Verification items for the finished model (mm, model axes). Face numbers are marked on the shaded views. A direction names the side the tool comes from. Round coordinates to 2 decimals unless told otherwise and drop trailing zeros. Order: outer loops, then holes, each group sorted by start corner. A loop starts at its lowest first (then second) coordinate and runs counter-clockwise, first axis right, second up. Notation, with made-up numbers: (54, 83) -> (81, 83) arc R30 ccw to (81, 113) -> close; hole circle Ø3 at (45.25, 49.25). An arc over 180 degrees is marked (long way). Put each result on its own line as item: value.
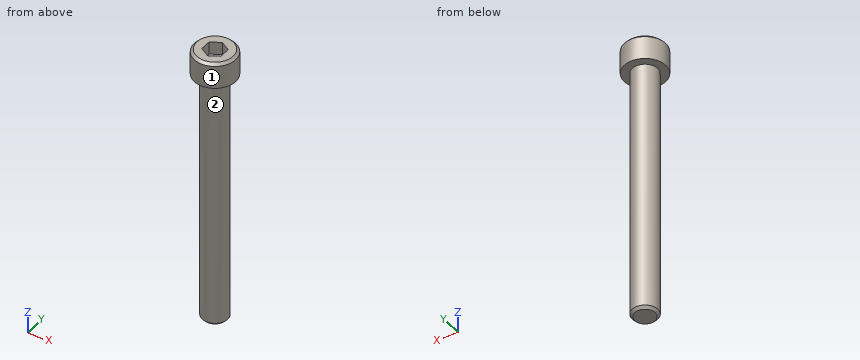
Autodesk Inventor part; units mm, degrees
ref_plane "YZ Plane" through (0, 0, 0) normal (1, 0, 0) x (0, 1, 0)
ref_plane "XZ Plane" through (0, 0, 0) normal (0, 1, 0) x (-1, 0, 0)
ref_plane "XY Plane" through (0, 0, 0) normal (0, 0, 1) x (1, 0, 0)
sketch "Sketch1" plane through (0, 0, 0) normal (0, 0, 1) x (1, 0, 0)
  circle A0 centre (0, 0) radius 4
  dimension "Diameter" = 8
extrude "Extrusion1" add sketch "Sketch1" along normal blind 80
sketch "Sketch2" plane through (0, 0, 80) normal (0, 0, 1) x (1, 0, 0)
  circle A0 centre (0, 0) radius 4
  circle A1 centre (0, 0) radius 6.5
  dimension "Head_Diameter" = 13
extrude "Extrusion2" add sketch "Sketch2" along normal blind 8 contours A0 | A1
sketch "Sketch3" plane through (0, 0, 88) normal (0, 0, 1) x (1, 0, 0)
  circle A0 centre (0, 0) radius 6.5
  circle A1 centre (0, 0) radius 3.4641 construction
  line L0 (0, 3.4641) -> (3, 1.7321)
  line L1 (3, -1.7321) -> (3, 1.7321)
  line L2 (0, 3.4641) -> (-3, 1.7321)
  line L3 (-3, -1.7321) -> (-3, 1.7321)
  line L4 (-3, -1.7321) -> (0, -3.4641)
  line L5 (3, -1.7321) -> (0, -3.4641)
  dimension "Hex_Width" = 6
extrude "Extrusion3" cut sketch "Sketch3" against normal blind 4 contours L0 L1 L5 L4 L3 L2
thread "Thread1"
chamfer "Chamfer1" distance 0.8 angle 45 2 edges at (-6.5, 0, 88) (-4, 0, 0)
equation "\"d9\" = ThreadLength"
equation "\"d12\" = Chamfer"
equation "\"ThreadLength\" = 28"
properties part number "SCREW,SOCKET HD,P,12.9,M8X1.25X80MM"
Item 1: Sectioned sample at A-A, the plane y = 0. Record the boundary of the cut face in (x, z).
Geometry check:
outline: (-6.5, 80) -> (-4, 80) -> (-4, 0.8) -> (-3.2, 0) -> (3.2, 0) -> (4, 0.8) -> (4, 80) -> (6.5, 80) -> (6.5, 87.2) -> (5.7, 88) -> (3, 88) -> (3, 84) -> (-3, 84) -> (-3, 88) -> (-5.7, 88) -> (-6.5, 87.2) -> close
Item 2: Sectioned sample at B-B, the plane z = 8.5. Record the boundary of the cut face in (x, y), then the cut area to 3 significant figures.
Geometry check:
outline: circle Ø8 at (0, 0)
area: 50.3 mm2
Item 3: Material ranges on line 1 along Z through (x, y) = (-3, -3.75); line 2 along Z through (x, y) = (0.75, 1); line 3 along X through (y, z) = (0.25, 83), recorded low to high.
Geometry check:
line 1: 80 to 88
line 2: 0 to 84
line 3: -6.5 to 6.5
Item 4: Tool access check on the marked faces 1 and 2. Record the directions out of +Z, -Z, +X, -X, +Y, -Y that give a thin tool (end or side, any length) a straight path to the whole face; none if there is none.
Geometry check:
face 1: +Z, -Z
face 2: -Z
Item 5: Depth check by flat-ended pin: pin 1 Ø4 at (y, z) = (0.5, 27) entering from -X; pin 2 Ø2 at (y, z) = (-3, 14.5) entering from -X; pin 3 Ø1.8 at (x, y) = (1, -1) entering from +Z. Enter the tip coordinate at first touch or a pass-through.
Geometry check:
pin 1: x = -4
pin 2: x = -3.46
pin 3: z = 84
